from build123d import *

# Parameters (mm, degrees)
SKETCH_W        = 29
SKETCH_H        = 29
PAD_DEPTH       = 15
SKETCH001_R     = 13.8
POCKET_DEPTH    = 15
SKETCH003_W     = 4
SKETCH003_H     = 15
PAD001_DEPTH    = 5
SKETCH005_W     = 2
SKETCH005_H     = 9.016475
POCKET001_DEPTH = 15
SKETCH006_R     = 1.241628
POCKET002_DEPTH = 5
SKETCH007_W     = 2
SKETCH007_H     = 15
PAD002_DEPTH    = 5
SKETCH008_W     = 2
SKETCH008_H     = 15
PAD003_DEPTH    = 5
SKETCH009_R     = 1.7
POCKET003_DEPTH = 5


with BuildPart() as part:
    # Sketch → Pad (new body)
    with BuildSketch(Plane.XY):
        Rectangle(SKETCH_W, SKETCH_H)
    extrude(amount=PAD_DEPTH)

    # Sketch001 (on Face6 of Pad) → Pocket (cut)
    with BuildSketch(Plane.XY.offset(15)):
        Circle(SKETCH001_R)
    extrude(amount=-POCKET_DEPTH, mode=Mode.SUBTRACT)

    # Sketch003 (on Face1 of Pocket) → Pad001 (join)
    with BuildSketch(Plane(origin=(0, 14.5, 0), x_dir=(-1, 0, 0), z_dir=(0, 1, 0))):
        with Locations((0, 7.5)):
            Rectangle(SKETCH003_W, SKETCH003_H)
    extrude(amount=PAD001_DEPTH)

    # Sketch005 (on Face11 of Pad001) → Pocket001 (cut)
    with BuildSketch(Plane.XY.offset(15)):
        with Locations((0, 17.054208)):
            Rectangle(SKETCH005_W, SKETCH005_H)
    extrude(amount=-POCKET001_DEPTH, mode=Mode.SUBTRACT)

    # Sketch006 (on Face3 of Pocket001) → Pocket002 (cut)
    with BuildSketch(Plane(origin=(-2, 0, 0), x_dir=(0, -1, 0), z_dir=(-1, 0, 0))):
        with Locations((-17.992161, 7.5)):
            Circle(SKETCH006_R)
    extrude(amount=-POCKET002_DEPTH, mode=Mode.SUBTRACT)

    # Sketch007 (on Face1 of Pocket002) → Pad002 (join)
    with BuildSketch(Plane(origin=(0, 14.5, 0), x_dir=(-1, 0, 0), z_dir=(0, 1, 0))):
        with Locations((13.5, 7.5)):
            Rectangle(SKETCH007_W, SKETCH007_H)
    extrude(amount=PAD002_DEPTH)

    # Sketch008 (on Face7 of Pad002) → Pad003 (join)
    with BuildSketch(Plane.XZ.offset(14.5)):
        with Locations((-13.5, 7.5)):
            Rectangle(SKETCH008_W, SKETCH008_H)
    extrude(amount=PAD003_DEPTH)

    # Sketch009 (on Face26 of Pad003) → Pocket003 (cut)
    with BuildSketch(Plane(origin=(-14.5, 0, 0), x_dir=(0, -1, 0), z_dir=(-1, 0, 0))):
        with Locations((-17, 7.453879)):
            Circle(SKETCH009_R)
        with Locations((17, 7.453879)):
            Circle(SKETCH009_R)
    extrude(amount=-POCKET003_DEPTH, mode=Mode.SUBTRACT)


solid = part.part
Can you work these out from the model? Positions are in its coordinate system, mm. A direction names the side the tool comes from. Round coordinates to 2 decimals unless told otherwise and drop trailing zeros. Write each loop counter-clockwise with the first axis right and the second up, starting at its lowest first coordinate (ties: lowest second). Pieces come first, ordered by that corner, then holes. Notation, with made-up numbers: (-5.5, 30.25) -> (45.5, 30.25) arc R16 ccw to (45.5, 60.25) -> close; hole circle Ø1 at (-18.5, -17.5). An arc over 180 degrees is marked (long way). One line per question, with ' | ' between items. Start each with the question number.
1) If we mould it in two halves opening along X, with no side actions, what happens to faces 1 (the cylindrical face through (-13.51, -18.57, 6.8)), 2 (the flat face through (-12.5, -15, 7)), 3 (the flat face through (-7, 14.5, 7))? For each: released by +X, released by -X, zero draft, split by the parting line, or undercut.
2) Suppose I cut it at D-D on z = 7. Count the separate pieces of the cut face and the enclosed holes in it, then the cut area to 3 significant figures.
3) Suppose I cut it at A-A on x = -1.5. Write out the boundary of the cut face in (y, z).
4) On a 3-axis mill with a long thin cutter (end or side, diameter ignored), from which of +Z, -Z, +X, -X, +Y, -Y can I reach the whole of each face in a straight line? I mean faces 4 (the cylindrical face through (1.493, 16.808, 7.873)), 5 (the flat face through (8, 14.5, 7)), 6 (the flat face through (1, 16.6, 7.6)), 7 (the flat face through (1, -14.5, 7)), 8 (the cylindrical face through (-13.514, 15.379, 7.965)). Say none if no direction works.
5) Suppose I cut it at B-B on y = -17. Write out the boundary of the cut face in (x, z), then the cut area to 3 significant figures.
6) Suppose I cut it at C-C on z = 2.75. Write out the boundary of the cut face in (x, y), then the cut area to 3 significant figures.
7) I'm going to push flat-ended pins straight in: P1, Ø1.5, axis at y = -16.5, z = 5.5, coming from the +X side; P2, Ø2, axis at x = 1, z = 4, coming from the -Y side; P3, Ø2.5, axis at y = 17.5, z = 5.5, coming from the +X side. Where does each tip first touch, or does it pass through?
8) I need wall thicknesses on line 1 (X direction, y = 17, z = 12.5); line 2 (X direction, y = 14, z = 8.5); line 3 (X direction, y = 7.5, z = 5.25). Which ranges of each line are inside material? Lowest first, please. Write a range as [from, to].
Return value:
1) face 1: zero draft | face 2: released by +X | face 3: undercut
2) separate pieces: 5 | enclosed holes: 0 | area: 254 mm2
3) outline: (-14.5, 0) -> (-13.72, 0) -> (-13.72, 15) -> (-14.5, 15) -> close; (13.72, 0) -> (19.5, 0) -> (19.5, 15) -> (13.72, 15) -> close; hole circle Ø2.48 at (17.99, 7.5)
4) face 4: +X | face 5: +Z, -Z, +X, +Y | face 6: +Z, -Z, +Y | face 7: +Z, -Z, +X, -Y | face 8: -X
5) outline: (-14.5, 0) -> (-12.5, 0) -> (-12.5, 5.75) -> (-14.5, 5.75) -> close; (-14.5, 9.15) -> (-12.5, 9.15) -> (-12.5, 15) -> (-14.5, 15) -> close | area: 23.2 mm2
6) outline: (-14.5, -19.5) -> (-12.5, -19.5) -> (-12.5, -14.5) -> (14.5, -14.5) -> (14.5, 14.5) -> (2, 14.5) -> (2, 19.5) -> (1, 19.5) -> (1, 13.76) arc R13.8 cw (long way) to (-1, 13.76) -> (-1, 19.5) -> (-2, 19.5) -> (-2, 14.5) -> (-12.5, 14.5) -> (-12.5, 19.5) -> (-14.5, 19.5) -> close | area: 271 mm2
7) P1: stops at x = -12.5 | P2: stops at y = -14.5 | P3: stops at x = 2
8) line 1: x = [-14.5, -12.5], [-2, -1], [1, 2] | line 2: x = [-14.5, -1], [1, 14.5] | line 3: x = [-14.5, -11.58], [11.58, 14.5]
